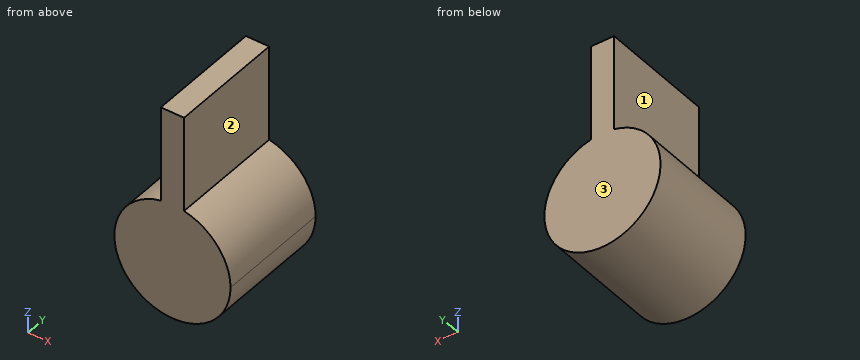
from build123d import *

# Parameters (mm, degrees)
F1_DEPTH = 25.4
F2_DEPTH = 25.4


with BuildPart() as f1:
    # F0 (on Front) → F1 (new body)
    with BuildSketch(Plane.XZ):
        with BuildLine():
            ThreePointArc((-2.54, 12.443408), (-8.032185, -9.837378), (12.7, 0))
            ThreePointArc((12.7, 0), (9.837378, 8.032185), (2.54, 12.443408))
            Line((2.54, 12.443408), (2.54, 0))
            Line((2.54, 0), (-2.54, 0))
            Line((-2.54, 0), (-2.54, 12.443408))
        make_face()
    extrude(amount=F1_DEPTH)

    # F0 (on Front) → F2 (join, through all)
    with BuildSketch(Plane.XZ):
        with BuildLine():
            ThreePointArc((-2.54, 12.443408), (0, 12.7), (2.54, 12.443408))
            Line((2.54, 12.443408), (2.54, 33.27414))
            Line((2.54, 33.27414), (-2.54, 33.27414))
            Line((-2.54, 33.27414), (-2.54, 12.443408))
        make_face()
        with BuildLine():
            Line((2.54, 0), (2.54, 12.443408))
            ThreePointArc((2.54, 12.443408), (0, 12.7), (-2.54, 12.443408))
            Line((-2.54, 12.443408), (-2.54, 0))
            Line((-2.54, 0), (2.54, 0))
        make_face()
    extrude(amount=F2_DEPTH)


solid = f1.part
Model file for the job. Use its own axes, mm. Face numbers are marked on the shaded views. A direction names the side the tool comes from. Round coordinates to 2 decimals unless told otherwise and drop trailing zeros. Order: outer loops, then holes, each group sorted by start corner. A loop starts at its lowest first (then second) coordinate and runs counter-clockwise, first axis right, second up.
(1) Pin check, flat tips, straight feed: pin 1 (2 mm diameter, centred on x = 7, y = -9, fed in from -Z); pin 2 (6 mm diameter, centred on y = -8.5, z = 18.5, fed in from +X); pin 3 (6 mm diameter, centred on x = 8.5, y = -9, fed in from -Z); pin 4 (5 mm diameter, centred on x = -6.5, z = 22, fed in from -Y). Stop position of each tip, or through.
(2) Band-saw the part on A-A (y = -10.5). List the corners of the cut face in (x, z).
(3) Band-saw the part on B-B (z = 29). List the corners of the cut face in (x, y), then the cut area to 3 significant figures.
(4) Drill centre lines: line 1 (Z direction, x = -0.5, y = -11.5); line 2 (X direction, y = -20, z = 21); line 3 (Z direction, x = -6.75, y = -18). Where is each one in solid material? Low to high.
(5) Band-saw the part on C-C (x = 8). List the corners of the cut face in (y, z).
(6) 3-axis set-ups, long thin cutter, end or side, ignore diameter. For the marked faces 1, 2 and 3: which of +Z, -Z, +X, -X, +Y, -Y reach the whole face in a straight line?
Verdict:
1. pin 1: stops at z = -11.19
1. pin 2: stops at x = 2.54
1. pin 3: stops at z = -11.45
1. pin 4: passes through
2. outline: (-2.54, 12.44) arc R12.7 ccw (long way) to (2.54, 12.44) - (2.54, 33.27) - (-2.54, 33.27) - close
3. outline: (-2.54, -25.4) - (2.54, -25.4) - (2.54, 0) - (-2.54, 0) - close
3. area: 129 mm2
4. line 1: z = -12.69 to 33.27
4. line 2: x = -2.54 to 2.54
4. line 3: z = -10.76 to 10.76
5. outline: (-25.4, -9.86) - (0, -9.86) - (0, 9.86) - (-25.4, 9.86) - close
6. face 1: +Z, -X, +Y, -Y
6. face 2: +Z, +X, +Y, -Y
6. face 3: +Z, -Z, +X, -X, +Y
